Read the model definition and answer for the solid it produces. Units are mm, in the model's axes. Give positions to 0.01 mm unless a question says otherwise; leave off trailing zeros. Write each loop counter-clockwise with the first axis right and the second up, starting at its lowest first coordinate (ties: lowest second). Pieces come first, ordered by that corner, then holes. Notation, with made-up numbers: (49.25, 78.25) -> (86.25, 78.25) arc R32 ccw to (86.25, 115.25) -> close; hole circle Ø3 at (37, 88.5). An arc over 180 degrees is marked (long way). Answer as CSV lines item,"result". Start each with the question number.
1. Find the intervals of material crossed by line 1 (Y direction, x = 202, z = -380), in increasing order.
2. The part is cut by section A-A, the plane x = 291. Determine the outline of the cut face in (y, z).
3. The part is cut by section C-C, the plane x = 200. Determine the outline of the cut face in (y, z).
4. The part is cut by section B-B, the plane z = -661.5. Determine the outline of the cut face in (x, y).
5. For a pull along Y with two mould halves and no side action, classify faces 1 (the conical face through (213.61, -30, -500.6)), 2 (the flat face through (153, 0, -507)), 3 (the flat face through (197, 20, -507)), 4 (the flat face through (197, 10, 0)) as pulls with the +Y half, pulls with the -Y half, needs draft (parallel to the pull), parting line crosses it, or undercut.
6. Given pin 1 (8 mm diameter, centred on x = 349, z = -706, fed in from -Y), flat-ended and moving along its own axis, determine where the tip first touches the part or whether it passes through.
from build123d import *

# Parameters (mm, degrees)
SCHIZZO1_W                   = 400
SCHIZZO1_H                   = 1000
ESTRUSIONE_ESTRUSIONE1_DEPTH = 20
SCHIZZO2_R                   = 20
ESTRUSIONE_ESTRUSIONE2_DEPTH = 50
ESTRUSIONE_ESTRUSIONE2_TAPER = 12


with BuildPart() as part:
    # Schizzo1 → Estrusione-Estrusione1 (new body)
    with BuildSketch(Plane(origin=(0, 0, 0), x_dir=(1, 0, 0), z_dir=(0, 1, 0))):
        with Locations((200, 500)):
            Rectangle(SCHIZZO1_W, SCHIZZO1_H)
    extrude(amount=ESTRUSIONE_ESTRUSIONE1_DEPTH)

    # Schizzo2 → Estrusione-Estrusione2 (add)
    with BuildSketch(Plane(origin=(0, 0, 0), x_dir=(-1, 0, 0), z_dir=(0, -1, 0))):
        with Locations((-200, 500)):
            Circle(SCHIZZO2_R)
    extrude(amount=ESTRUSIONE_ESTRUSIONE2_DEPTH, taper=ESTRUSIONE_ESTRUSIONE2_TAPER)

    # Schizzo4 → Rivoluzione1 (revolve)
    with BuildSketch(Plane(origin=(200, 0, 0), x_dir=(0, 0, -1), z_dir=(1, 0, 0))):
        with BuildLine():
            Line((485, -60), (515, -60))
            ThreePointArc((515, -60), (500, -45), (485, -60))
        make_face()
    revolve(axis=Axis((200, -60, -485), (0, 0, -1)))


solid = part.part
Results found:
1,line 1,"y = 0 to 20"
2,outline,"(0, -1000) -> (20, -1000) -> (20, 0) -> (0, 0) -> close"
3,outline,"(-48.54, -509.68) -> (0, -520) -> (0, -1000) -> (20, -1000) -> (20, 0) -> (0, 0) -> (0, -480) -> (-48.54, -490.32) arc R15 ccw (long way) to start"
4,outline,"(0, 0) -> (400, 0) -> (400, 20) -> (0, 20) -> close"
5,face 1,"undercut"
5,face 2,"pulls with the -Y half"
5,face 3,"pulls with the +Y half"
5,face 4,"needs draft"
6,pin 1,"stops at y = 0"
